Geometry: see drawing. Coordinates: mm, zero at the bounding-box minimum. A direction names the side the tool comes from. Give positions to 0.01 mm unless a question says otherwise; leave off trailing zeros. Write each loop counter-clockwise with the first axis right and the second up, starting at its lowest first coordinate (ties: lowest second). Pieces come first, ordered by that corner, then holes. Notation, with made-up numbers: M 73,83.25 L 119,83.25 A19 ccw 119,118.25 Z; hole C 13,-14 d8. An arc over 180 degrees is marked long. Use a Markdown table: item, result. Add a question column.
1) Draft query along Y for the marked faces 3, 4 and 5. Return one class per face: +Y half, -Y half, draft (parallel to the pull), parting line (faces both ways), or undercut.
2) Section A-A on x = 15. Return the cut outline in (y, z), then the cut area to 3 significant figures.
3) Set-up query: the marked faces 1 and 2. Return all of +Z, -Z, +X, -X, +Y, -Y with unobstructed straight access to the full face (end or side cutting, diameter ignored); none if empty.
4) Pin query (flat end, axial travel): pin 1 (8 mm diameter, centred on x = 15, y = 15, fed in from +Z); pin 2 (3 mm diameter, centred on y = 4, z = 1.5, fed in from -X). Return the tip coordinate at first contact, or that it passes through.
5) Section C-C on z = 3.5. Return the cut outline in (x, y).
6) Section D-D on z = 1.85. Return the cut outline in (x, y), then the cut area to 3 significant figures.
7) Line query: line 1 (Y direction, x = 15, z = 1.9); line 2 (Y direction, x = 15, z = 3.8); line 3 (Z direction, x = 14, y = 26). Output: solid intervals per line, ascending.
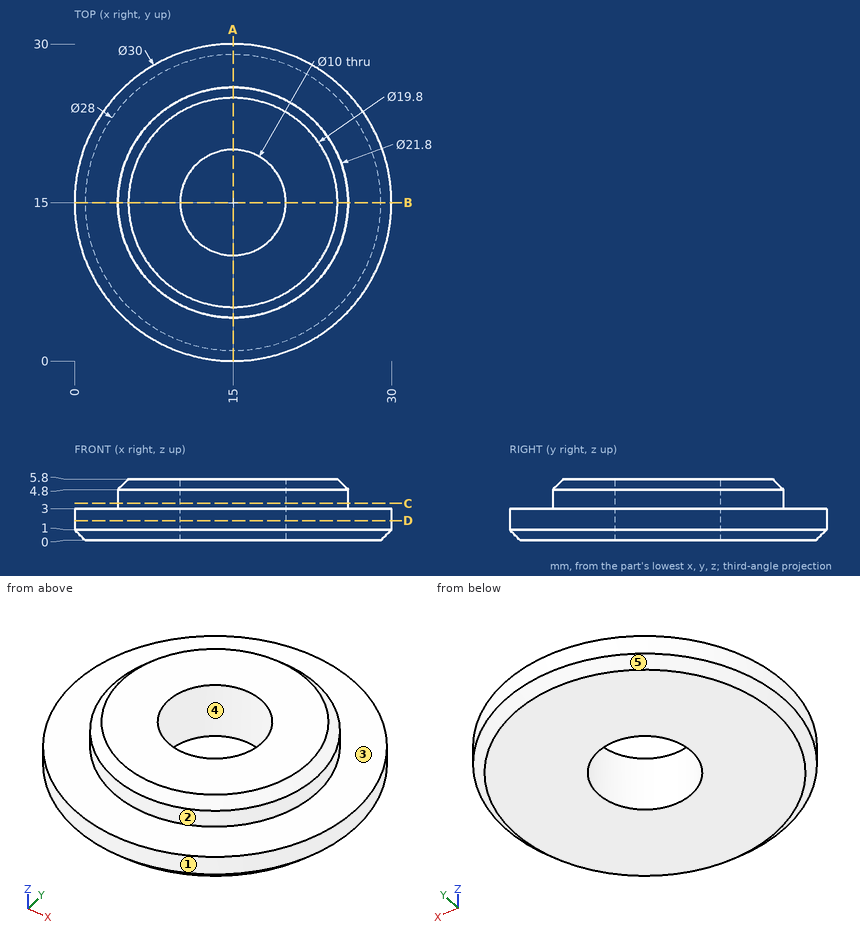
Found:
| question | item | result |
|---|---|---|
| 1 | face 3 | draft |
| 1 | face 4 | undercut |
| 1 | face 5 | parting line |
| 2 | outline | M 0,1 L 1,0 L 10,0 L 10,5.8 L 5.1,5.8 L 4.1,4.8 L 4.1,3 L 0,3 Z; M 20,0 L 29,0 L 30,1 L 30,3 L 25.9,3 L 25.9,4.8 L 24.9,5.8 L 20,5.8 Z |
| 2 | area | 91.0 mm² |
| 3 | face 1 | +Z, -Z |
| 3 | face 2 | +Z |
| 4 | pin 1 | through |
| 4 | pin 2 | x = 3.39 |
| 5 | outline | C 15,15 d21.8; hole C 15,15 d10 |
| 6 | outline | C 15,15 d30; hole C 15,15 d10 |
| 6 | area | 628 mm² |
| 7 | line 1 | 0 to 10, 20 to 30 |
| 7 | line 2 | 4.1 to 10, 20 to 25.9 |
| 7 | line 3 | 0 to 3 |
